Check sheet for the drawn part. Datum: minimum x, y, z corner. Units: mm. Coordinates: 2 decimals unless noted, no trailing zeros. Loops run counter-clockwise (first coordinate to the right, second up) from the corner with the lowest first, then second, coordinate; pieces in that order, holes last.
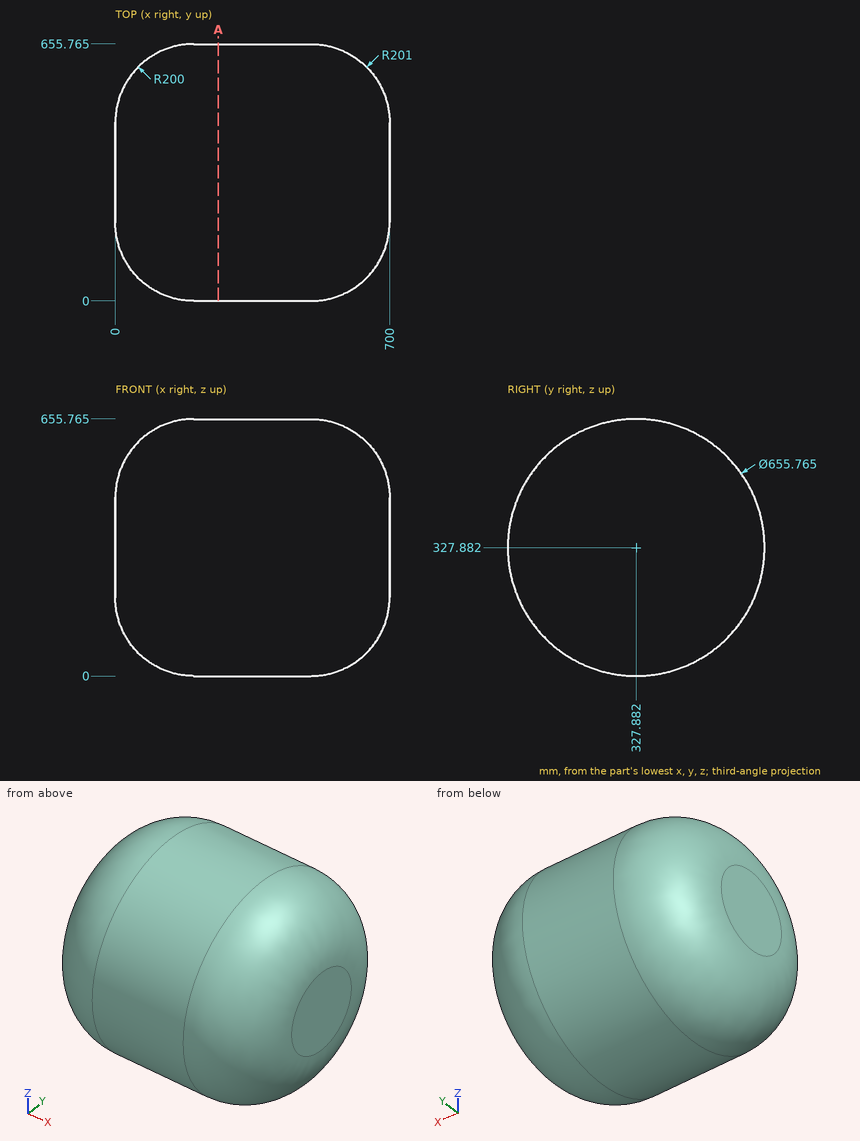
(1) Scan lines: L1, parallel to Z at x = 456, y = 321.5; L2, parallel to X at y = 190, z = 410 (1 decimal); L3, parallel to Z at x = 304, y = 586 (1 decimal). Record each from-to range of solid material in increasing order.
Findings:
L1: z = 0.06 to 655.7
L2: x = 2.7 to 697.2
L3: z = 125.7 to 530.1
(2) Gauge pin test, flat ends, axial feed: pin 1 Ø2 at (x, y) = (96.5, 215) entering from -Z; pin 2 Ø1 at (x, z) = (140.5, 521.5) entering from +Y (1 decimal); pin 3 Ø12 at (x, z) = (185, 518) entering from +Y. Record the tip position at first contact, or that the pin passes through.
Findings:
pin 1: stops at z = 50.22
pin 2: stops at y = 581.6
pin 3: stops at y = 598.54
(3) Sectioned sample at A-A on x = 263. Record the cut outline in (y, z) (1 decimal).
Findings:
outline: circle Ø655.8 at (327.9, 327.9)
